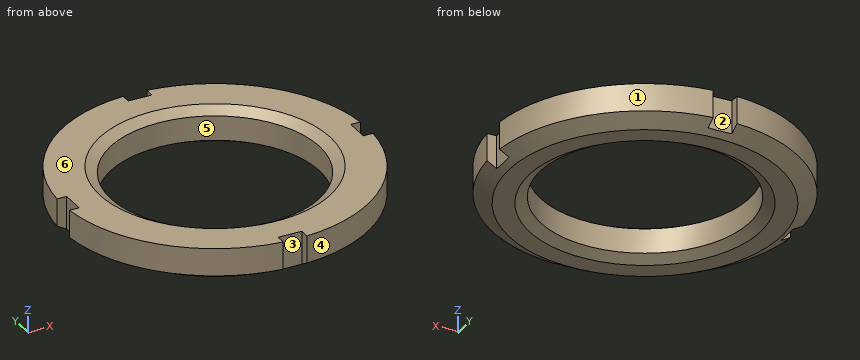
```python
from build123d import *

# Parameters (mm, degrees)
SKICA1_R                 = 90
SKICA1_R_2               = 61.6
VYSUNOUT1_DEPTH          = 11
ZKOSIT2_SIZE             = 3.74
ZKOSIT2_SIZE2            = 6.47787002
ZKOSIT3_SIZE             = 3.74
ZKOSIT3_SIZE2            = 6.47787002
ODEBRAT_VYSUNUT_M1_REACH = 131.167
SKICA2_W                 = 14
SKICA2_H                 = 6
KRUHOV_POLE1_COUNT       = 4


with BuildPart() as part:
    # Skica1 → Vysunout1 (new, symmetric)
    with BuildSketch(Plane.XY):
        Circle(SKICA1_R)
        Circle(SKICA1_R_2, mode=Mode.SUBTRACT)
    extrude(amount=VYSUNOUT1_DEPTH, both=True)

    # Zkosit2
    zkosit2_edges = [part.edges().sort_by_distance(p)[0] for p in [
        (-61.6, 0, -11),
    ]]
    zkosit2_side = [part.faces().sort_by_distance(p)[0] for p in [
        (-61.6, 0, 0),
    ]]
    chamfer(zkosit2_edges, length=ZKOSIT2_SIZE, length2=ZKOSIT2_SIZE2, reference=zkosit2_side[0])

    # Zkosit3
    zkosit3_edges = [part.edges().sort_by_distance(p)[0] for p in [
        (-61.6, 0, 11),
    ]]
    zkosit3_side = [part.faces().sort_by_distance(p)[0] for p in [
        (-61.6, 0, 1.87),
    ]]
    chamfer(zkosit3_edges, length=ZKOSIT3_SIZE, length2=ZKOSIT3_SIZE2, reference=zkosit3_side[0])

    # Skica4 → Odebrat otočením1 (revolve, cut)
    with BuildSketch(Plane(origin=(0, 0, 0), x_dir=(1, 0, 0), z_dir=(0, 1, 0))):
        Polygon((90, 11), (80, 11), (90, 5.226497308), align=None)
    revolve(axis=Axis((0, 0, 0), (0, 0, -1)), mode=Mode.SUBTRACT)

    # Odebrat vysunutím1: up to this cone (the profile starts inside it)
    odebrat_vysunut_m1_end = Plane(origin=(0, 0, 11), z_dir=(0, 0, 1)).offset(-68.188020535) * Cone(1.732e-06, 550.723116052, 317.960138302, align=(Align.CENTER, Align.CENTER, Align.MIN), mode=Mode.PRIVATE)
    # Skica2 → Odebrat vysunutím1 (cut, up to the surface)
    with BuildSketch(Plane.XY.offset(11), mode=Mode.PRIVATE) as odebrat_vysunut_m1_sk1:
        with Locations((0, 87)):
            Rectangle(SKICA2_W, SKICA2_H)
    odebrat_vysunut_m1_tool1 = extrude(odebrat_vysunut_m1_sk1.sketch, amount=-ODEBRAT_VYSUNUT_M1_REACH, mode=Mode.PRIVATE) & odebrat_vysunut_m1_end
    odebrat_vysunut_m1 = odebrat_vysunut_m1_tool1.solids().sort_by_distance((0, 87, 11))[0]
    add(odebrat_vysunut_m1, mode=Mode.SUBTRACT)

    # Kruhové pole1: Odebrat vysunutím1 ×4 about axis
    kruhov_pole1_axis = Axis((0, 0, 0), (0, 0, 1))
    for i in range(1, KRUHOV_POLE1_COUNT):
        add(odebrat_vysunut_m1.rotate(kruhov_pole1_axis, i * 360 / KRUHOV_POLE1_COUNT), mode=Mode.SUBTRACT)


solid = part.part
```
Geometry check sheet. Reference: the model listing, model coordinates, mm. Face numbers are marked on the shaded views. A direction names the side the tool comes from. Coordinates: 2 decimals unless noted, no trailing zeros. Order: outer loops, then holes, each group sorted by start corner. A loop starts at its lowest first (then second) coordinate and runs counter-clockwise, first axis right, second up. Notation, with made-up numbers: (-35.75, -23.75) - (22.25, -23.75) arc R29 ccw to (22.25, 13.25) - close; hole circle Ø1 at (43, -16.5). An arc over 180 degrees is marked (long way). Answer as a JSON object with one key per item and string values. Group by question number.
Item 1: Sectioned sample at C-C, the plane z = 2.25. Record the cut outline in (x, y), and give its area (3 significant figures).
Item 2: Draft check along X on the marked faces 3, 4, 5 and 6. Enter one of: +X half, -X half, draft (parallel to the pull), parting line (faces both ways), or undercut.
Item 3: Scan lines: probe 1 along Y at (x, z) = (0, 2.75); probe 2 along Y at (x, z) = (-53, 3); probe 3 along X at (y, z) = (17.5, -2). Record each from-to range of solid material in increasing order.
Item 4: Tool access check on the marked faces 1 and 2. Record the directions out of +Z, -Z, +X, -X, +Y, -Y that give a thin tool (end or side, any length) a straight path to the whole face; none if there is none.
Item 5: Depth check by flat-ended pin: pin 1 Ø6.5 at (y, z) = (85.5, -1.5) entering from +X; pin 2 Ø1.5 at (x, z) = (-8.5, -1.5) entering from -Y; pin 3 Ø1 at (x, z) = (-14.5, -9) entering from -Y. Enter the tip coordinate at first touch or a pass-through.
Item 6: Sectioned sample at A-A, the plane y = 0. Record the cut outline in (x, z).
Resolved:
{
 "1": {"outline": "(-89.73, -7) arc R90 ccw to (-7, -89.73) - (-7, -84) - (7, -84) - (7, -89.73) arc R90 ccw to (89.73, -7) - (84, -7) - (84, 7) - (89.73, 7) arc R90 ccw to (7, 89.73) - (7, 84) - (-7, 84) - (-7, 89.73) arc R90 ccw to (-89.73, 7) - (-84, 7) - (-84, -7) - close; hole circle Ø123.2 at (0, 0)", "area": "13,200 mm^2"},
 "2": {"face 3": "undercut", "face 4": "+X half", "face 5": "undercut", "face 6": "draft"},
 "3": {"probe 1": "-84 to -61.6, 61.6 to 84", "probe 2": "-72.74 to -31.39, 31.39 to 72.74", "probe 3": "-88.28 to -59.06, 59.06 to 88.28"},
 "4": {"face 1": "+Z, -Z, +X, +Y", "face 2": "+Z, -Z, +Y"},
 "5": {"pin 1": "x = 36.54", "pin 2": "y = -89.67", "pin 3": "y = -83.08"},
 "6": {"outline": "(-84, -8.69) - (-80, -11) - (-68.08, -11) - (-61.6, -7.26) - (-61.6, 7.26) - (-68.08, 11) - (-84, 11) - close; (61.6, -7.26) - (68.08, -11) - (80, -11) - (84, -8.69) - (84, 11) - (68.08, 11) - (61.6, 7.26) - close"}
}
